from build123d import *

# Parameters (mm, degrees)
F0_W     = 9.32
F0_H     = 45.13
F0_R     = 1.5
F1_DEPTH = 6
F3_DEPTH = 9.32


with BuildPart() as f1:
    # F0 (on Top) → F1 (new body)
    with BuildSketch(Plane.XY):
        Rectangle(F0_W, F0_H)
        with Locations((0, -18.065)):
            Circle(F0_R, mode=Mode.SUBTRACT)
        with Locations((0, -11.065)):
            Circle(F0_R, mode=Mode.SUBTRACT)
        with Locations((0, 11.065)):
            Circle(F0_R, mode=Mode.SUBTRACT)
        with Locations((0, 18.065)):
            Circle(F0_R, mode=Mode.SUBTRACT)
    extrude(amount=F1_DEPTH)

    # F2 (on face) → F3 (cut, through all)
    with BuildSketch(Plane.YZ.offset(4.66)):
        with BuildLine():
            ThreePointArc((1.1785714286, 3.9278843612), (1.4173667738, 3.490990253), (1.5, 3))
            Line((1.5, 3), (6, 3))
            ThreePointArc((6, 3), (3.9724555913, 5.4549512652), (1.1785714286, 3.9278843612))
        make_face()
        with BuildLine():
            ThreePointArc((1.5, 3), (1.4173667738, 2.509009747), (1.1785714286, 2.0721156388))
            ThreePointArc((1.1785714286, 2.0721156388), (3.9724555913, 0.5450487348), (6, 3))
            Line((6, 3), (1.5, 3))
        make_face()
        with BuildLine():
            Line((-6, 3), (-1.5, 3))
            ThreePointArc((-1.5, 3), (-1.4173667738, 3.490990253), (-1.1785714286, 3.9278843612))
            ThreePointArc((-1.1785714286, 3.9278843612), (-3.9724555913, 5.4549512652), (-6, 3))
        make_face()
        with BuildLine():
            ThreePointArc((-6, 3), (-3.9724555913, 0.5450487348), (-1.1785714286, 2.0721156388))
            ThreePointArc((-1.1785714286, 2.0721156388), (-1.4173667738, 2.509009747), (-1.5, 3))
            Line((-1.5, 3), (-6, 3))
        make_face()
        with BuildLine():
            Line((-1.5, 3), (-1, 3))
            ThreePointArc((-1, 3), (-1.0450487348, 3.4724555913), (-1.1785714286, 3.9278843612))
            ThreePointArc((-1.1785714286, 3.9278843612), (-1.4173667738, 3.490990253), (-1.5, 3))
        make_face()
        with BuildLine():
            ThreePointArc((-1.5, 3), (-1.4173667738, 2.509009747), (-1.1785714286, 2.0721156388))
            ThreePointArc((-1.1785714286, 2.0721156388), (-1.0450487348, 2.5275444087), (-1, 3))
            Line((-1, 3), (-1.5, 3))
        make_face()
        with BuildLine():
            Line((-1, 3), (0, 3))
            Line((0, 3), (0, 4.5))
            ThreePointArc((0, 4.5), (-0.6550471198, 4.3494121946), (-1.1785714286, 3.9278843612))
            ThreePointArc((-1.1785714286, 3.9278843612), (-1.0450487348, 3.4724555913), (-1, 3))
        make_face()
        with BuildLine():
            Line((0, 4.5), (0, 3))
            Line((0, 3), (1, 3))
            ThreePointArc((1, 3), (1.0450487348, 3.4724555913), (1.1785714286, 3.9278843612))
            ThreePointArc((1.1785714286, 3.9278843612), (0.6550471198, 4.3494121946), (0, 4.5))
        make_face()
        with BuildLine():
            ThreePointArc((1.1785714286, 3.9278843612), (1.0450487348, 3.4724555913), (1, 3))
            Line((1, 3), (1.5, 3))
            ThreePointArc((1.5, 3), (1.4173667738, 3.490990253), (1.1785714286, 3.9278843612))
        make_face()
        with BuildLine():
            ThreePointArc((1, 3), (1.0450487348, 2.5275444087), (1.1785714286, 2.0721156388))
            ThreePointArc((1.1785714286, 2.0721156388), (1.4173667738, 2.509009747), (1.5, 3))
            Line((1.5, 3), (1, 3))
        make_face()
        with BuildLine():
            Line((0, 3), (0, 1.5))
            ThreePointArc((0, 1.5), (0.6550471198, 1.6505878054), (1.1785714286, 2.0721156388))
            ThreePointArc((1.1785714286, 2.0721156388), (1.0450487348, 2.5275444087), (1, 3))
            Line((1, 3), (0, 3))
        make_face()
        with BuildLine():
            ThreePointArc((-1.1785714286, 2.0721156388), (-0.6550471198, 1.6505878054), (0, 1.5))
            Line((0, 1.5), (0, 3))
            Line((0, 3), (-1, 3))
            ThreePointArc((-1, 3), (-1.0450487348, 2.5275444087), (-1.1785714286, 2.0721156388))
        make_face()
    extrude(amount=-F3_DEPTH, mode=Mode.SUBTRACT)


solid = f1.part
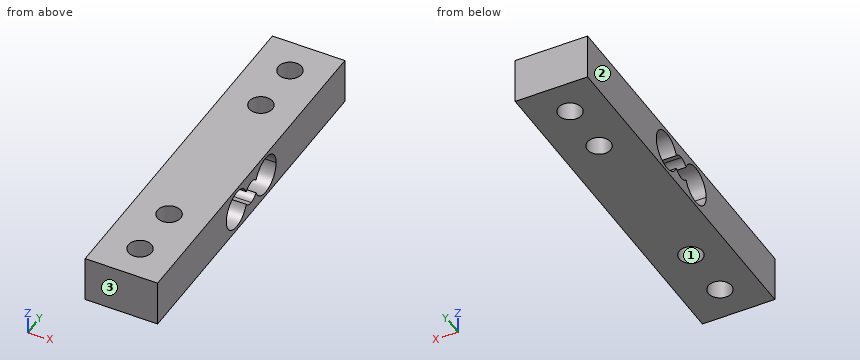
Work out the finished part from the listing and answer in its coordinate system (mm). Face numbers are marked on the shaded views. Round coordinates to 2 decimals unless told otherwise and drop trailing zeros. Order: outer loops, then holes, each group sorted by start corner. A loop starts at its lowest first (then second) coordinate and runs counter-clockwise, first axis right, second up. Notation, with made-up numbers: M -2.75,34.5 L 37.25,34.5 A27 cw 37.25,66.5 Z; hole C 26,60 d7. An arc over 180 degrees is marked long. Put each result on its own line as item: value. Start each with the question number.
Q1. For a pull along X with two mould halves and no side action, classify the marked faces 1, 2 and 3 as pulls with the +X half, pulls with the -X half, needs draft (parallel to the pull), parting line crosses it, or undercut.
Q2. Straight lines are drawn through the part: L1, parallel to Y at x = 0, z = 3.2 (3 decimals); L2, parallel to Z at x = 2.25, y = 1.5; L3, parallel to X at y = -11, z = 1.55. For each, find the intervals that lie inside material, in ascending order. Write a range as [from, to].
Q3. Section A-A, the plane x = 0 is taken. Write down the section's boundary in (y, z) (3 decimals).
Q4. Section B-B, the plane x = -3 is taken. Write down the section's boundary in (y, z) (3 decimals), and give its area (3 significant figures).
Q5. Section C-C, the plane y = -4 is taken. Write down the section's boundary in (x, z).
Findings below:
1. face 1: undercut
1. face 2: pulls with the -X half
1. face 3: needs draft
2. L1: y = [-22.565, -19.565], [-16.565, -12.565], [-9.565, -5.992], [5.992, 9.565], [12.565, 16.565], [19.565, 22.565]
2. L2: z = [0, 1.5], [4.5, 6]
2. L3: x = [-4.66, -1.5], [1.5, 4.66]
3. outline: M -22.565,0 L -19.565,0 L -19.565,6 L -22.565,6 Z; M -16.565,0 L -12.565,0 L -12.565,6 L -16.565,6 Z; M -9.565,0 L 9.565,0 L 9.565,6 L -9.565,6 Z; M 12.565,0 L 16.565,0 L 16.565,6 L 12.565,6 Z; M 19.565,0 L 22.565,0 L 22.565,6 L 19.565,6 Z; hole M -1.179,2.072 A1.5 ccw 1.179,2.072 A2.5 ccw long 1.179,3.928 A1.5 ccw -1.179,3.928 A2.5 ccw long Z
4. outline: M -22.565,0 L 22.565,0 L 22.565,6 L -22.565,6 Z; hole M -1.179,2.072 A1.5 ccw 1.179,2.072 A2.5 ccw long 1.179,3.928 A1.5 ccw -1.179,3.928 A2.5 ccw long Z
4. area: 226 mm^2
5. outline: M -4.66,0 L 4.66,0 L 4.66,0.55 L -4.66,0.55 Z; M -4.66,5.45 L 4.66,5.45 L 4.66,6 L -4.66,6 Z
